from build123d import *

# Parameters (mm, degrees)
SKETCH_1_R      = 0.6
EXTRUDE_1_DEPTH = 2


with BuildPart() as part:
    # 草图1 → 凸台-拉伸1 (new body)
    with BuildSketch(Plane(origin=(0, 0, 0), x_dir=(0, 0, -1), z_dir=(1, 0, 0))):
        Polygon((-5.483662069, -5.746212595), (22.48689596, 0.939195285), (21.934471639, 23.485878838), (17.91469757, 28.839240511), (8.158406363, 36.115117525), (0, 40.546620882), (-6.780914547, 43.602624476), (-13.936136859, 43.602624476), (-20.210913974, 40.546620882), (-34.455547379, 34.968652147), (-49.745371225, 33.281638151), (-2.678378839, 3.842593198), align=None)
        Circle(SKETCH_1_R, mode=Mode.SUBTRACT)
        with Locations((12.23711119, 0.518510559)):
            Circle(SKETCH_1_R, mode=Mode.SUBTRACT)
    extrude(amount=EXTRUDE_1_DEPTH)


solid = part.part
Input: part model. Units: mm. Frame: model coordinates. Give positions to 0.01 mm unless a question says otherwise; leave off trailing zeros. Write each loop counter-clockwise with the first axis right and the second up, starting at its lowest first coordinate (ties: lowest second). Pieces come first, ordered by that corner, then holes.
Q1. Section A-A, the plane x = 1.7. Output: boundary loops of the cut face in (y, z).
Q2. Pull-direction query (X, two-part tool) for faces 1 (the face through (0, 19, 6)), 2 (the face through (2, 19, 6)), 3 (the face through (0.99, -0.88, 4.06)); classes: pulls with the +X half, pulls with the -X half, needs draft (parallel to the pull), parting line crosses it, or undercut.
Q3. Section B-B, the plane z = 31. Output: boundary loops of the cut face in (x, y).
Q4. Section C-C, the plane y = 6. Output: boundary loops of the cut face in (x, z).
Q5. Material intervals for probe 1 along Y at (x, z) = (0.9, 0); probe 2 along Y at (x, z) = (0.5, 36.5); probe 3 along Z at (x, y) = (0.75, 30.5), sorted ascending.
Filled in:
1. outline: (-5.75, 5.48) - (0.94, -22.49) - (23.49, -21.93) - (28.84, -17.91) - (36.12, -8.16) - (40.55, 0) - (43.6, 6.78) - (43.6, 13.94) - (40.55, 20.21) - (34.97, 34.46) - (33.28, 49.75) - (3.84, 2.68) - close; hole circle Ø1.2 at (0, 0); hole circle Ø1.2 at (0.52, -12.24)
2. face 1: pulls with the -X half
2. face 2: pulls with the +X half
2. face 3: needs draft
3. outline: (0, 21.56) - (2, 21.56) - (2, 36.32) - (0, 36.32) - close
4. outline: (0, -22.36) - (2, -22.36) - (2, 6.13) - (0, 6.13) - close
5. probe 1: y = -4.44 to -0.6, 0.6 to 40.55
5. probe 2: y = 25 to 34.74
5. probe 3: z = -15.69 to 45.3
